Here's how the part is built. I have some questions about the finished solid (model axes, mm). A direction names the side the tool comes from. Round coordinates to 2 decimals unless told otherwise and drop trailing zeros. Loops run counter-clockwise (first coordinate to the right, second up) from the corner with the lowest first, then second, coordinate; pieces in that order, holes last. Notation, with made-up numbers: (48.5, 21.25) - (68.5, 21.25) arc R21 cw to (68.5, 46.25) - close; hole circle Ø7 at (-21, 49). An arc over 180 degrees is marked (long way). Answer as a JSON object with one key per item and string values. Group by question number.
1) Which directions (+Z, -Z, +X, -X, +Y, -Y) give clear straight access to the entire face, cutting with the end or side of a thin tool? Please do faces 1 (the face through (0, -10, -2)), 2 (the face through (10, 0, -2)).
2) I want a section at A-A, the plane y = 0. Please give me the cut outline in (x, z), then the cut area to 3 significant figures.
3) Will these pins go through, and if not, where does the flat tip stop? P1, Ø1.5, axis at y = -1, z = -3, coming from the +X side; P2, Ø1.5, axis at x = 35.5, z = -1.5, coming from the -Y side.
4) I want a section at D-D, the plane y = 36. Please give me the cut outline in (x, z).
5) If I drill on line 1 along Y through (x, z) = (0, -3.1); line 2 along Y through (x, z) = (50, -1.55); line 3 along X through (y, z) = (3.5, -3.25), over which ranges is the centre line in solid material (lowest first)? Write a range as [from, to].
6) I want a section at C-C, the plane z = -3.3. Please give me the cut outline in (x, y), then the cut area to 3 significant figures.
7) If we mould it in two halves opening along X, with no side actions, what happens to faces 3 (the face through (60, 36, -2)), 4 (the face through (-0.59, 4.46, -2.46)), 5 (the face through (52.08, 32.01, -2.46)), 6 (the face through (17, 25, 0))? For each: pulls with the +X half, pulls with the -X half, needs draft (parallel to the pull), parting line crosses it, or undercut.
8) I want a section at B-B, the plane x = 50. Please give me the cut outline in (y, z), then the cut area to 3 significant figures.
from build123d import *

# Parameters (mm, degrees)
SKETCH_1_R      = 4.5
EXTRUDE_1_DEPTH = 5
CHAMFER_1_SIZE  = 15


with BuildPart() as part:
    # 草图1 → 凸台-拉伸1 (new body)
    with BuildSketch(Plane.XY):
        Polygon((-10, 26), (-10, 10), (-10, -10), (10, -10), (10, 10), (10, 26), (40, 26), (60, 26), (60, 46), (40, 46), (10, 46), (-10, 46), align=None)
        Circle(SKETCH_1_R, mode=Mode.SUBTRACT)
        with Locations((0, 36)):
            Circle(SKETCH_1_R, mode=Mode.SUBTRACT)
        with Locations((50, 36)):
            Circle(SKETCH_1_R, mode=Mode.SUBTRACT)
    extrude(amount=-EXTRUDE_1_DEPTH)

    # 倒角1
    chamfer_1_edges = [part.edges().sort_by_distance(p)[0] for p in [
        (10, 26, -2.5),
    ]]
    chamfer(chamfer_1_edges, length=CHAMFER_1_SIZE)


solid = part.part
Outcome:
{
 "1": {"face 1": "+Z, -Z, +X, -X, -Y", "face 2": "+Z, -Z, +X, -Y"},
 "2": {"outline": "(-10, -5) - (-4.5, -5) - (-4.5, 0) - (-10, 0) - close; (4.5, -5) - (10, -5) - (10, 0) - (4.5, 0) - close", "area": "55.0 mm^2"},
 "3": {"P1": "x = 10", "P2": "y = 26"},
 "4": {"outline": "(-10, -5) - (-4.5, -5) - (-4.5, 0) - (-10, 0) - close; (4.5, -5) - (45.5, -5) - (45.5, 0) - (4.5, 0) - close; (54.5, -5) - (60, -5) - (60, 0) - (54.5, 0) - close"},
 "5": {"line 1": "[-10, -4.5], [4.5, 31.5], [40.5, 46]", "line 2": "[26, 31.5], [40.5, 46]", "line 3": "[-10, -2.83], [2.83, 10]"},
 "6": {"outline": "(-10, -10) - (10, -10) - (10, 11) - (25, 26) - (60, 26) - (60, 46) - (-10, 46) - close; hole circle Ø9 at (0, 0); hole circle Ø9 at (0, 36); hole circle Ø9 at (50, 36)", "area": "2,040 mm^2"},
 "7": {"face 3": "pulls with the +X half", "face 4": "undercut", "face 5": "undercut", "face 6": "needs draft"},
 "8": {"outline": "(26, -5) - (31.5, -5) - (31.5, 0) - (26, 0) - close; (40.5, -5) - (46, -5) - (46, 0) - (40.5, 0) - close", "area": "55.0 mm^2"}
}
